from build123d import *

# Parameters (mm, degrees)
F0_W     = 304.8
F0_H     = 609.6
F1_DEPTH = 1143
F2_T     = -12.7
F3_DEPTH = 12.701


with BuildPart() as f1:
    # F0 (on Top) → F1 (new body)
    with BuildSketch(Plane.XY):
        with Locations((152.4, -304.8)):
            Rectangle(F0_W, F0_H)
    extrude(amount=F1_DEPTH)

    # F2
    f2_openings = [f1.faces().sort_by_distance(p)[0] for p in [
        (152.4, -609.6, 571.5),
    ]]
    offset(amount=F2_T, openings=f2_openings)

    # F3 (cut, through all): a face of the model
    f3_faces = [f1.faces().sort_by_distance(p)[0] for p in [
        (152.4, -311.15, 12.7),
    ]]
    extrude(f3_faces, amount=-F3_DEPTH, mode=Mode.SUBTRACT)


solid = f1.part
Input: part model. Units: mm. Frame: model coordinates. A direction names the side the tool comes from. Coordinates: 2 decimals unless noted, no trailing zeros. Loops run counter-clockwise (first coordinate to the right, second up) from the corner with the lowest first, then second, coordinate; pieces in that order, holes last. Notation, with made-up numbers: (81, 86.25) -> (86, 86.25) arc R29 cw to (86, 110.25) -> close; hole circle Ø4 at (11.25, 18). An arc over 180 degrees is marked (long way). One line per item, written item: value.
(1) Cut plane A-A (z = 511.5). Output: boundary loops of the cut face in (x, y), then the cut area to 3 significant figures.
Answer below:
outline: (0, -609.6) -> (12.7, -609.6) -> (12.7, -12.7) -> (292.1, -12.7) -> (292.1, -609.6) -> (304.8, -609.6) -> (304.8, 0) -> (0, 0) -> close
area: 19,000 mm2
(2) Cut plane B-B (y = -99). Output: boundary loops of the cut face in (x, z), then the cut area to 3 significant figures.
Answer below:
outline: (0, 0) -> (12.7, 0) -> (12.7, 1130.3) -> (292.1, 1130.3) -> (292.1, 0) -> (304.8, 0) -> (304.8, 1143) -> (0, 1143) -> close
area: 32,600 mm2
(3) Draft query along X for faces 1 (the face through (150, 0, 563)), 2 (the face through (304.8, -309, 563)), 3 (the face through (154, -12.7, 573)), 4 (the face through (150, -307, 1130.3)). Return one class per face: pulls with the +X half, pulls with the -X half, needs draft (parallel to the pull), parting line crosses it, or undercut.
Answer below:
face 1: needs draft
face 2: pulls with the +X half
face 3: undercut
face 4: undercut
(4) Set-up query: faces 5 (the face through (5, -609.6, 569)), 6 (the face through (292.1, -315, 557)). Return all of +Z, -Z, +X, -X, +Y, -Y with unobstructed straight access to the full face (end or side cutting, diameter ignored); none if empty.
Answer below:
face 5: +Z, -Z, +X, -X, -Y
face 6: -Z, -Y
(5) Pin query (flat end, axial travel): pin 1 Ø5 at (x, y) = (255.5, -184.5) entering from -Z; pin 2 Ø6 at (x, z) = (153, 291) entering from -Y. Return the tip coordinate at first contact, or that it passes through.
Answer below:
pin 1: stops at z = 1130.3
pin 2: stops at y = -12.7
(6) Cut plane C-C (x = 117). Output: boundary loops of the cut face in (y, z), then the cut area to 3 significant figures.
Answer below:
outline: (-609.6, 1130.3) -> (-12.7, 1130.3) -> (-12.7, 0) -> (0, 0) -> (0, 1143) -> (-609.6, 1143) -> close
area: 22,100 mm2
(7) Ray query, line 1 along X through (y, z) = (-421, 107); line 2 along Y through (x, z) = (235, 695.5); line 3 along Z through (x, y) = (87, -484). Return the intervals inside material, ascending.
Answer below:
line 1: x = 0 to 12.7, 292.1 to 304.8
line 2: y = -12.7 to 0
line 3: z = 1130.3 to 1143
